Source: CAD feature listing. Evaluate the final solid. Frame: model axes, mm. A direction names the side the tool comes from. Give positions to 0.01 mm unless a question says otherwise; leave off trailing zeros. Order: outer loops, then holes, each group sorted by start corner. A loop starts at its lowest first (then second) coordinate and runs counter-clockwise, first axis right, second up.
1) Draft query along Z for faces 1 (the face through (7.841, -19.084, 21.446)), 2 (the face through (0, -20, 21.7)), 3 (the face through (-10, 14, 10.2)). Return one class per face: released by +Z, released by -Z, zero draft, split by the parting line, or undercut.
2) First-contact query: P1, Ø4, axis at x = 8, z = 10.5, coming from the +Y side; P2, Ø1, axis at x = 10, z = 8.5, coming from the -Y side; P3, Ø10, axis at x = 7.5, y = -22, coming from the +Z side. Flat tips, straight axial feed; report the tip coordinate or a pass-through.
3) Section C-C, the plane z = 18. Return loops of the section in (x, y).
4) Section D-D, the plane y = 15.5. Return loops of the section in (x, z), plus the area to 3 significant figures.
5) Section B-B, the plane x = 11.5. Return loops of the section in (y, z).
6) Material intervals for line 1 (Z direction, x = 17.5, y = 10.5); line 2 (Y direction, x = -13.5, z = 3.75); line 3 (Y direction, x = -4.5, z = 5.25), sorted ascending.
7) Access query for faces 4 (the face through (-8, -18.8, 21.4)), 5 (the face through (0, 0, 0)), 6 (the face through (-15, 14, 8)). Directions: +Z, -Z, +X, -X, +Y, -Y. A direction counts if a zero-diameter tool reaches every point of the face in a straight line with its end or side. Return the directions, or none.
8) Section A-A, the plane y = 0. Return loops of the section in (x, z), plus the area to 3 significant figures.
```python
from build123d import *

# Parameters (mm, degrees)
F0_R      = 19.75
F1_DEPTH  = 8
F2_R      = 21.425
F3_DEPTH  = 2.2
F4_R      = 16.2
F5_DEPTH  = 12
F10_DEPTH = 0.5


# Not quite as in the source:
# - the program builds the solid bodies; features that only make, move or delete a surface that nothing else refers to are left out


with BuildPart() as f1:
    # F0 (on Top) → F1 (new body)
    with BuildSketch(Plane.XY):
        Circle(F0_R)
    extrude(amount=F1_DEPTH)

    # F2 (on face) → F3 (join)
    with BuildSketch(Plane.XY.offset(8)):
        with Locations((-0.6810527993, 0.7295852411)):
            Circle(F2_R)
    extrude(amount=F3_DEPTH)

    # F4 (on face) → F5 (join)
    with BuildSketch(Plane.XY.offset(10.2)):
        Circle(F4_R)
    extrude(amount=F5_DEPTH)

    # F7 (on offset) → F10 (join)
    with BuildSketch(Plane.XY.offset(21.2)):
        with BuildLine():
            ThreePointArc((14.1136150197, -7.9527272727), (15.6697250027, -4.1109267009), (16.2, 0))
            ThreePointArc((16.2, 0), (-4.1109267009, 15.6697250027), (-14.1136150197, -7.9527272727))
            ThreePointArc((-14.1136150197, -7.9527272727), (0, -16.2), (14.1136150197, -7.9527272727))
        make_face()
        with BuildLine():
            ThreePointArc((14.1136150197, -7.9527272727), (0, -16.2), (-14.1136150197, -7.9527272727))
            Line((-14.1136150197, -7.9527272727), (-1.7424216074, -29.9077441077))
            ThreePointArc((-1.7424216074, -29.9077441077), (0, -30.9259259259), (1.7424216074, -29.9077441077))
            Line((1.7424216074, -29.9077441077), (14.1136150197, -7.9527272727))
        make_face()
    extrude(amount=F10_DEPTH)


solid = f1.part
```
From the geometry:
1. face 1: zero draft
1. face 2: released by +Z
1. face 3: undercut
2. P1: stops at y = 21.08
2. P2: stops at y = -18.12
2. P3: stops at z = 21.7
3. outline: circle Ø32.4 at (0, 0)
4. outline: (-16.2, 8) - (-12.24, 8) - (-12.24, 0) - (12.24, 0) - (12.24, 8) - (14.84, 8) - (14.84, 10.2) - (4.71, 10.2) - (4.71, 22.2) - (-4.71, 22.2) - (-4.71, 10.2) - (-16.2, 10.2) - close
4. area: 377 mm2
5. outline: (-16.9, 8) - (-16.06, 8) - (-16.06, 0) - (16.06, 0) - (16.06, 8) - (18.35, 8) - (18.35, 10.2) - (11.41, 10.2) - (11.41, 22.2) - (-11.41, 22.2) - (-11.41, 21.7) - (-12.59, 21.7) - (-12.59, 21.2) - (-11.41, 21.2) - (-11.41, 10.2) - (-16.9, 10.2) - close
6. line 1: z = 8 to 10.2
6. line 2: y = -14.42 to 14.42
6. line 3: y = -19.23 to 19.23
7. face 4: +Z, -X, -Y
7. face 5: -Z, +X, -X, +Y, -Y
7. face 6: -Z
8. outline: (-22.09, 8) - (-19.75, 8) - (-19.75, 0) - (19.75, 0) - (19.75, 8) - (20.73, 8) - (20.73, 10.2) - (16.2, 10.2) - (16.2, 22.2) - (-16.2, 22.2) - (-16.2, 10.2) - (-22.09, 10.2) - close
8. area: 799 mm2
